Here's how the part is built. I have some questions about the finished solid (model axes, mm). A direction names the side the tool comes from. Coordinates: 2 decimals unless noted, no trailing zeros. Write each loop counter-clockwise with the first axis right and the second up, starting at its lowest first coordinate (ties: lowest second). Pieces come first, ordered by that corner, then holes. Notation, with made-up numbers: M -1.5,80 L 55.5,80 A16 ccw 55.5,106 Z; hole C -5.5,85 d11. An arc over 180 degrees is marked long. Use one line per item in the form item = value. Start each with the question number.
1. I'm going to push flat-ended pins straight in: pin 1 Ø8 at (x, z) = (-3, 37.5) entering from -Y; pin 2 Ø1 at (x, z) = (11, 90) entering from +Y; pin 3 Ø1 at (y, z) = (6.5, 24) entering from +X; pin 4 Ø1 at (y, z) = (-2, 94) entering from -X. Where does each tip first touch, or does it pass through?
2. I want a section at A-A, the plane x = 0. List the corners of the cut face in (y, z) for me.
3. I want a section at C-C, the plane y = 3.5. List the corners of the cut face in (x, z) for me, plus the area to 3 significant figures.
4. Please list where these lines run through material, in increasing order: line 1 along Y through (x, z) = (-0.5, 161); line 2 along X through (y, z) = (9, 146); line 3 along Y through (x, z) = (0, 73). Write a range as [from, to].
5. I want a section at D-D, the plane z = 63. List the corners of the cut face in (x, y) for me, plus the area to 3 significant figures.
6. On a 3-axis mill with a long thin cutter (end or side, diameter ignored), from which of +Z, -Z, +X, -X, +Y, -Y can I reach the whole of each face in a straight line? I mean faces 4 (the face through (-5, 9, 0)), 5 (the face through (0.8, 10.4, 145)). Say none if no direction works.
7. Thinking about a two-plate mould opening in Y: for faces 1 (the face through (-2.17, -9.76, 88.74)), 2 (the face through (-5, 9, 180)), 3 (the face through (-2.601, -11.715, 88.74)), which applies, released by +Y, released by -Y, zero draft, split by the parting line, or undercut?
8. I want a section at B-B, the plane y = -7.5. List the corners of the cut face in (x, z) for me, plus the area to 3 significant figures.
from build123d import *

# Parameters (mm, degrees)
SCHIZZO1_R                    = 12
SCHIZZO1_R_2                  = 10
ESTRUSIONE_ESTRUSIONE1_DEPTH  = 180
SCHIZZO2_W                    = 115
SCHIZZO2_H                    = 12
TAGLIO_ESTRUSIONE1_DEPTH      = 20
TAGLIO_ESTRUSIONE1_DEPTH_BACK = 20


with BuildPart() as part:
    # Schizzo1 → Estrusione-Estrusione1 (new body)
    with BuildSketch(Plane.XY):
        Circle(SCHIZZO1_R)
        Circle(SCHIZZO1_R_2, mode=Mode.SUBTRACT)
    extrude(amount=ESTRUSIONE_ESTRUSIONE1_DEPTH)

    # Schizzo2 → Taglio-Estrusione1 (cut, two sides)
    with BuildSketch(Plane(origin=(0, 0, 0), x_dir=(0, 0, -1), z_dir=(1, 0, 0))) as taglio_estrusione1_sk:
        with Locations((-87.5, 6)):
            Rectangle(SCHIZZO2_W, SCHIZZO2_H)
    extrude(amount=TAGLIO_ESTRUSIONE1_DEPTH, mode=Mode.SUBTRACT)
    extrude(taglio_estrusione1_sk.sketch, amount=-TAGLIO_ESTRUSIONE1_DEPTH_BACK, mode=Mode.SUBTRACT)


solid = part.part
Answer list:
q1.pin_1 = -12
q1.pin_2 = 0
q1.pin_3 = 10.39
q1.pin_4 = -11.91
q2.outline = M -12,0 L -10,0 L -10,180 L -12,180 Z; M 10,0 L 12,0 L 12,30 L 10,30 Z; M 10,145 L 12,145 L 12,180 L 10,180 Z
q3.outline = M -11.48,0 L -9.37,0 L -9.37,30 L -11.48,30 Z; M -11.48,145 L -9.37,145 L -9.37,180 L -11.48,180 Z; M 9.37,0 L 11.48,0 L 11.48,30 L 9.37,30 Z; M 9.37,145 L 11.48,145 L 11.48,180 L 9.37,180 Z
q3.area = 274 mm²
q4.line_1 = [-11.99, -9.99], [9.99, 11.99]
q4.line_2 = [-7.94, -4.36], [4.36, 7.94]
q4.line_3 = [-12, -10]
q5.outline = M -12,0 A12 ccw 12,0 L 10,0 A10 cw -10,0 Z
q5.area = 69.1 mm²
q6.face_4 = -Z, +X, -X, +Y, -Y
q6.face_5 = +X, -X, +Y
q7.face_1 = undercut
q7.face_2 = zero draft
q7.face_3 = split by the parting line
q8.outline = M -9.37,0 L -6.61,0 L -6.61,180 L -9.37,180 Z; M 6.61,0 L 9.37,0 L 9.37,180 L 6.61,180 Z
q8.area = 991 mm²
